from build123d import *

# Parameters (mm, degrees)
BODY_DEPTH                    = 6.35
HANDLE_DEPTH                  = 6.35
SKETCH11_R                    = 5
LOCKING_MECHANISM_HOLES_DEPTH = 6.36
FILLET1_R                     = 40
FILLET2_R                     = 40
SKETCH12_W                    = 304.8
SKETCH12_H                    = 50.8
BOSS_EXTRUDE1_DEPTH           = 12.7
CUT_EXTRUDE3_DEPTH            = 12.7


with BuildPart() as part:
    # Sketch1 → Body (new body)
    with BuildSketch(Plane(origin=(0, 0, 0), x_dir=(1, 0, 0), z_dir=(0, 1, 0))):
        Polygon((0, 0), (294, 0), (336.996020767, 43.003978862), (336.996020767, 337.003978862), (217, 456.999999629), (77, 456.999999629), (-42.996020767, 337.003978862), (-42.996020767, 43.003978862), align=None)
    extrude(amount=BODY_DEPTH)

    # Sketch2 → Handle (cut)
    with BuildSketch(Plane(origin=(0, 6.35, 0), x_dir=(1, 0, 0), z_dir=(0, 1, 0))):
        with BuildLine():
            Line((112.35, 441.799999629), (181.65, 441.799999629))
            ThreePointArc((181.65, 441.799999629), (197.5, 425.949999629), (181.65, 410.099999629))
            Line((181.65, 410.099999629), (112.35, 410.099999629))
            ThreePointArc((112.35, 410.099999629), (96.5, 425.949999629), (112.35, 441.799999629))
        make_face()
    extrude(amount=-HANDLE_DEPTH, mode=Mode.SUBTRACT)

    # Sketch11 → Locking Mechanism Holes (cut)
    with BuildSketch(Plane(origin=(0, 6.35, 0), x_dir=(1, 0, 0), z_dir=(0, 1, 0))):
        with Locations(Location((221.65, 421.999999629, 0), (0, 0, 270))):
            Circle(SKETCH11_R)
        with Locations(Location((72.35, 421.999999629, 0), (0, 0, 270))):
            Circle(SKETCH11_R)
    extrude(amount=-LOCKING_MECHANISM_HOLES_DEPTH, mode=Mode.SUBTRACT)

    # Fillet1
    fillet1_edges = [part.edges().sort_by_distance(p)[0] for p in [
        (77, 3.175, -456.999999629),
        (217, 3.175, -456.999999629),
    ]]
    fillet(fillet1_edges, radius=FILLET1_R)

    # Fillet2
    fillet2_edges = [part.edges().sort_by_distance(p)[0] for p in [
        (-42.996020767, 3.175, -43.003978862),
        (-42.996020767, 3.175, -337.003978862),
        (336.996020767, 3.175, -337.003978862),
        (336.996020767, 3.175, -43.003978862),
        (294, 3.175, 0),
        (0, 3.175, 0),
    ]]
    fillet(fillet2_edges, radius=FILLET2_R)

    # Sketch12 → Boss-Extrude1 (add)
    with BuildSketch(Plane.XZ):
        with Locations((147, -190.5)):
            Rectangle(SKETCH12_W, SKETCH12_H)
    extrude(amount=BOSS_EXTRUDE1_DEPTH)

    # Sketch13 → Cut-Extrude3 (cut)
    with BuildSketch(Plane.XZ.offset(12.7)):
        with BuildLine():
            Line((261.3, -203.2), (32.7, -203.2))
            ThreePointArc((32.7, -203.2), (20, -190.5), (32.7, -177.8))
            Line((32.7, -177.8), (261.3, -177.8))
            ThreePointArc((261.3, -177.8), (274, -190.5), (261.3, -203.2))
        make_face()
    extrude(amount=-CUT_EXTRUDE3_DEPTH, mode=Mode.SUBTRACT)


solid = part.part
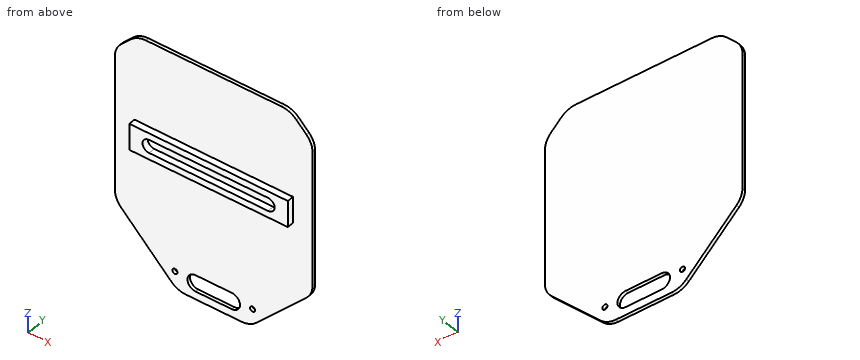
Geometry check sheet. Reference: the model listing, model coordinates, mm. Give positions to 0.01 mm unless a question says otherwise; leave off trailing zeros. Order: outer loops, then holes, each group sorted by start corner. A loop starts at its lowest first (then second) coordinate and runs counter-clockwise, first axis right, second up.
1. Depth check by flat-ended pin: pin 1 (6.5 mm diameter, centred on x = 101.5, y = -3.5, fed in from +Z); pin 2 (10 mm diameter, centred on y = -5.5, z = -180, fed in from +X); pin 3 (16 mm diameter, centred on x = 221.65, z = -422, fed in from -Y). Enter the tip coordinate at first touch or a pass-through.
Completed:
pin 1: stops at z = -165.1
pin 2: stops at x = 299.4
pin 3: stops at y = 0
2. Sectioned sample at C-C (z = -422). Record the boundary of the cut face in (x, y).
Completed:
outline: (42, 0) - (67.35, 0) - (67.35, 6.35) - (42, 6.35) - close; (77.35, 0) - (97, 0) - (97, 6.35) - (77.35, 6.35) - close; (197, 0) - (216.65, 0) - (216.65, 6.35) - (197, 6.35) - close; (226.65, 0) - (252, 0) - (252, 6.35) - (226.65, 6.35) - close
3. Scan lines: line 1 (X direction, y = 2.25, z = -422); line 2 (Y direction, x = 150.5, z = -283.5); line 3 (X direction, y = -6, z = -185). Record each from-to range of solid material in increasing order.
Completed:
line 1: x = 42 to 67.35, 77.35 to 97, 197 to 216.65, 226.65 to 252
line 2: y = 0 to 6.35
line 3: x = -5.4 to 21.25, 272.75 to 299.4
4. Sectioned sample at D-D (x = 221.65). Record the boundary of the cut face in (y, z), then the cut area to 3 significant figures.
Completed:
outline: (-12.7, -215.9) - (0, -215.9) - (0, -417) - (6.35, -417) - (6.35, 0) - (0, 0) - (0, -165.1) - (-12.7, -165.1) - (-12.7, -177.8) - (0, -177.8) - (0, -203.2) - (-12.7, -203.2) - close; (0, -450.91) - (6.35, -450.91) - (6.35, -427) - (0, -427) - close
area: 3,120 mm2
5. Sectioned sample at B-B (x = 44). Record the boundary of the cut face in (y, z).
Completed:
outline: (-12.7, -215.9) - (0, -215.9) - (0, -424) - (6.35, -424) - (6.35, 0) - (0, 0) - (0, -165.1) - (-12.7, -165.1) - (-12.7, -177.8) - (0, -177.8) - (0, -203.2) - (-12.7, -203.2) - close
6. Sectioned sample at A-A (y = -7.5). Record the boundary of the cut face in (x, z).
Completed:
outline: (-5.4, -215.9) - (299.4, -215.9) - (299.4, -165.1) - (-5.4, -165.1) - close; hole (32.7, -203.2) - (261.3, -203.2) arc R12.7 ccw to (261.3, -177.8) - (32.7, -177.8) arc R12.7 ccw to start
